Build history of the part. All positions in model axes, mm. Face numbers are marked on the shaded views. A direction names the side the tool comes from. Round coordinates to 2 decimals unless told otherwise and drop trailing zeros. Write each loop counter-clockwise with the first axis right and the second up, starting at its lowest first coordinate (ties: lowest second). Pieces come first, ordered by that corner, then holes. Notation, with made-up numbers: (87, 69.25) - (99, 69.25) arc R22 ccw to (99, 108.25) - close; hole circle Ø8 at (67.5, 6). An arc over 180 degrees is marked (long way). Write each question's results on one line, items separated by ' | '.
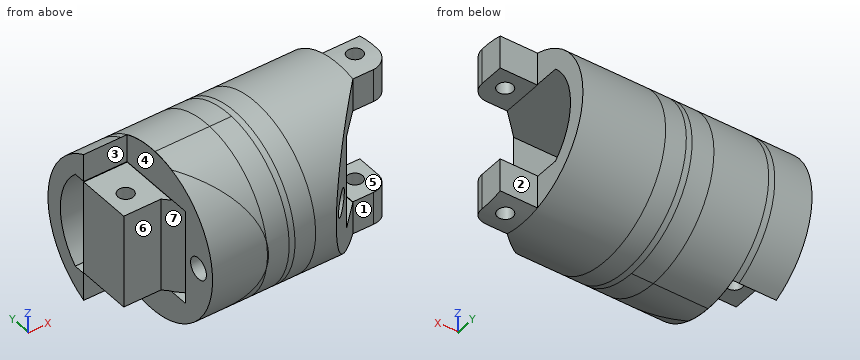
from build123d import *
from build123d.topology import SkipClean

# Parameters (mm, degrees)
SKETCH1_R           = 10
BOSS_EXTRUDE1_DEPTH = 10
SKETCH4_R           = 1.305
CUT_EXTRUDE3_DEPTH  = 25.5
BOSS_EXTRUDE2_START = 4.5
BOSS_EXTRUDE2_DEPTH = 4.5
SKETCH6_R           = 0.935
CUT_EXTRUDE4_DEPTH  = 12.25
SKETCH7_W           = 11.364916732
SKETCH7_H           = 5
BOSS_EXTRUDE3_DEPTH = 4.5
SKETCH8_R           = 0.935
CUT_EXTRUDE5_DEPTH  = 7.25
BOSS_EXTRUDE4_DEPTH = 4.5
CUT_EXTRUDE6_START  = -0.75
CUT_EXTRUDE6_DEPTH  = 0.75
SKETCH12_W          = 5.25
SKETCH12_H          = 4
CUT_EXTRUDE7_DEPTH  = 1.6
CUT_EXTRUDE8_DEPTH  = 15.8
FILLET1_R           = 2
CUT_EXTRUDE9_DEPTH  = 10.8
SKETCH15_W          = 11.364916732
SKETCH15_H          = 6.6
CUT_EXTRUDE10_DEPTH = 1.6
CUT_EXTRUDE11_DEPTH = 15
BOSS_EXTRUDE5_REACH = 35.438
SKETCH17_R          = 10
SKETCH17_R_2        = 1.305
CUT_EXTRUDE12_DEPTH = 14
SCALE1_SCALE        = 0.8


with BuildPart() as part:
    # Sketch1 → Boss-Extrude1 (new, symmetric)
    with BuildSketch(Plane(origin=(0, 0, 0), x_dir=(0, 0, -1), z_dir=(1, 0, 0))):
        Circle(SKETCH1_R)
    extrude(amount=BOSS_EXTRUDE1_DEPTH, both=True)

    # Sketch4 → Cut-Extrude3 (cut, symmetric)
    with BuildSketch(Plane(origin=(0, -0.76336978, 0), x_dir=(0, 0, -1), z_dir=(1, 0, 0))):
        with Locations((0, -6.913267104)):
            Circle(SKETCH4_R)
    extrude(amount=CUT_EXTRUDE3_DEPTH, both=True, mode=Mode.SUBTRACT)

    # Sketch5 → Boss-Extrude2 (add)
    with BuildSketch(Plane(origin=(10, 0, 0), x_dir=(0, 0, -1), z_dir=(1, 0, 0)).offset(BOSS_EXTRUDE2_START)):
        with BuildLine():
            Line((-9.682458366, -2.5), (-5.682458366, -2.5))
            Line((-5.682458366, -2.5), (-5.682458366, 2.5))
            Line((-5.682458366, 2.5), (-9.682458366, 2.5))
            ThreePointArc((-9.682458366, 2.5), (-10, 0), (-9.682458366, -2.5))
        make_face()
    boss_extrude2 = extrude(amount=-BOSS_EXTRUDE2_DEPTH)

    # Mirror1: Boss-Extrude2 across plane
    add(boss_extrude2.mirror(Plane.XY))

    # Sketch6 → Cut-Extrude4 (cut, symmetric)
    with SkipClean():  # the faces are left unmerged after this step: merging them gives an invalid solid
        with BuildSketch(Plane.XY):
            with Locations((12.25, 0.25)):
                Circle(SKETCH6_R)
        extrude(amount=CUT_EXTRUDE4_DEPTH, both=True, mode=Mode.SUBTRACT)

    # Sketch7 → Boss-Extrude3 (add)
    with SkipClean():  # the faces are left unmerged after this step: merging them gives an invalid solid
        with BuildSketch(Plane.ZY.offset(10)):
            Rectangle(SKETCH7_W, SKETCH7_H)
        extrude(amount=BOSS_EXTRUDE3_DEPTH)

    # Sketch8 → Cut-Extrude5 (cut, symmetric)
    with SkipClean():  # the faces are left unmerged after this step: merging them gives an invalid solid
        with BuildSketch(Plane.XY):
            with Locations((-12.25, 0.25)):
                Circle(SKETCH8_R)
        extrude(amount=CUT_EXTRUDE5_DEPTH, both=True, mode=Mode.SUBTRACT)

    # Sketch10 → Boss-Extrude4 (add)
    with SkipClean():  # the faces are left unmerged after this step: merging them gives an invalid solid
        with BuildSketch(Plane.ZY.offset(10)):
            with BuildLine():
                Line((9.682458366, 2.5), (-9.682458366, 2.5))
                ThreePointArc((-9.682458366, 2.5), (0, 10), (9.682458366, 2.5))
            make_face()
        extrude(amount=BOSS_EXTRUDE4_DEPTH)

    # Cut-Extrude6: read off the stored shape, not the designer's step
    # Cut-Extrude6 outline → Cut-Extrude6 (cut)
    with SkipClean():  # the faces are left unmerged after this step: merging them gives an invalid solid
        with BuildSketch(Plane.ZY.offset(10).offset(CUT_EXTRUDE6_START)):
            with BuildLine():
                ThreePointArc((-9.682458366, 2.5), (-9.369942303, -3.493448331), (-5.682458366, -8.228588392))
                Line((-5.682458366, -8.228588392), (-5.682458366, 2.5))
                Line((-5.682458366, 2.5), (-9.682458366, 2.5))
            make_face()
            with BuildLine():
                Line((5.682458366, 2.5), (5.682458366, -8.228588392))
                ThreePointArc((5.682458366, -8.228588392), (9.369942303, -3.493448331), (9.682458366, 2.5))
                Line((9.682458366, 2.5), (5.682458366, 2.5))
            make_face()
        extrude(amount=CUT_EXTRUDE6_DEPTH, mode=Mode.SUBTRACT)

    # Sketch12 → Cut-Extrude7 (cut)
    with SkipClean():  # the faces are left unmerged after this step: merging them gives an invalid solid
        with BuildSketch(Plane.XZ.offset(-2.5)):
            with Locations((-11.875, -7.682458366)):
                Rectangle(SKETCH12_W, SKETCH12_H)
            with Locations((-11.875, 7.682458366)):
                Rectangle(SKETCH12_W, SKETCH12_H)
        extrude(amount=-CUT_EXTRUDE7_DEPTH, mode=Mode.SUBTRACT)

    # Sketch13 → Cut-Extrude8 (cut, symmetric)
    with SkipClean():  # the faces are left unmerged after this step: merging them gives an invalid solid
        with BuildSketch(Plane.XY):
            Polygon((-10, -8.228588392), (-10, -2.5), (-2.5, -10), (-10, -10), align=None)
        extrude(amount=CUT_EXTRUDE8_DEPTH, both=True, mode=Mode.SUBTRACT)

    # Fillet1
    fillet1_edges = [part.edges().sort_by_distance(p)[0] for p in [
        (14.5, -2.5, 7.682458366),
        (14.5, -2.5, -7.682458366),
    ]]
    fillet(fillet1_edges, radius=FILLET1_R)

    # Sketch14 → Cut-Extrude9 (cut, symmetric)
    with SkipClean():  # the faces are left unmerged after this step: merging them gives an invalid solid
        with BuildSketch(Plane.XY):
            Polygon((10, -10), (10, -2.5), (2.5, -10), align=None)
        extrude(amount=CUT_EXTRUDE9_DEPTH, both=True, mode=Mode.SUBTRACT)

    # Sketch15 → Cut-Extrude10 (cut)
    with SkipClean():  # the faces are left unmerged after this step: merging them gives an invalid solid
        with BuildSketch(Plane(origin=(10, 0, 0), x_dir=(0, 0, -1), z_dir=(1, 0, 0))):
            with Locations((0, -0.8)):
                Rectangle(SKETCH15_W, SKETCH15_H)
        extrude(amount=-CUT_EXTRUDE10_DEPTH, mode=Mode.SUBTRACT)

    # Sketch16 → Cut-Extrude11 (cut)
    with SkipClean():  # the faces are left unmerged after this step: merging them gives an invalid solid
        with BuildSketch(Plane(origin=(10, 0, 0), x_dir=(0, 0, -1), z_dir=(1, 0, 0))):
            with BuildLine():
                Line((-5.75, 5.5), (-5.75, -5.5))
                Line((-5.75, -5.5), (5.75, -5.5))
                Line((5.75, -5.5), (5.75, 5.5))
                ThreePointArc((5.75, 5.5), (0, 7.956915231), (-5.75, 5.5))
            make_face()
        extrude(amount=-CUT_EXTRUDE11_DEPTH, mode=Mode.SUBTRACT)


with BuildPart() as body_2:
    # Split1: the piece on the far side of the plane
    add(part.part)
    split(bisect_by=Plane(origin=(0, 0, 0), x_dir=(0, 0, 1), z_dir=(1, 0, 0)), keep=Keep.BOTTOM)


with BuildPart() as part_1:
    add(part.part)

    # Split1
    split(bisect_by=Plane(origin=(0, 0, 0), x_dir=(0, 0, 1), z_dir=(1, 0, 0)), keep=Keep.TOP)


with BuildPart() as part_2:
    # Body-Move/Copy1: moved
    add(part_1.part.moved(Location((15.8, 0, 0))))


    # Sketch17 → Boss-Extrude5 (add, up to next)
    with BuildSketch(Plane.ZY.offset(-15.8), mode=Mode.PRIVATE) as boss_extrude5_sk1:
        with Locations(Location((0, 0, 0), (0, 0, 357.134016017))):
            Circle(SKETCH17_R)
        with Locations(Location((0, -7.676636884, 0), (0, 0, 180))):
            Circle(SKETCH17_R_2, mode=Mode.SUBTRACT)
        with BuildLine():
            Line((-5.75, -5.5), (5.75, -5.5))
            Line((5.75, -5.5), (5.75, 5.5))
            ThreePointArc((5.75, 5.5), (0, 7.956915231), (-5.75, 5.5))
            Line((-5.75, 5.5), (-5.75, -5.5))
        make_face(mode=Mode.SUBTRACT)
    boss_extrude5_tool1 = extrude(boss_extrude5_sk1.sketch, amount=BOSS_EXTRUDE5_REACH, mode=Mode.PRIVATE) - body_2.part
    add(boss_extrude5_tool1.solids().sort_by_distance((15.8, 0.485858, -9.705003))[0])


with BuildPart() as body_2_1:
    # Body-Move/Copy2: moved
    add(body_2.part.moved(Location((9.26, 0, 0))))

    # Combine4: union part
    add(part_2.part)

    # Sketch18 → Cut-Extrude12 (cut)
    with SkipClean():  # the faces are left unmerged after this step: merging them gives an invalid solid
        with BuildSketch(Plane.ZY.offset(5.24)):
            with BuildLine():
                Line((-5.75, 5.5), (-5.75, 4.1))
                Line((-5.75, 4.1), (5.75, 4.1))
                Line((5.75, 4.1), (5.75, 5.5))
                ThreePointArc((5.75, 5.5), (0, 7.956915231), (-5.75, 5.5))
            make_face()
        extrude(amount=-CUT_EXTRUDE12_DEPTH, mode=Mode.SUBTRACT)


with BuildPart() as body_2_2:
    # Scale1: scaled about (10.157754057, 0.26372377, 1.86e-07)
    add(body_2_1.part.scale(SCALE1_SCALE).moved(Location((2.031550811, 0.052744754, 3.7e-08))))


with BuildPart() as body_2_2_1:
    # Split2: the piece on the far side of the plane
    add(body_2_2.part)
    split(bisect_by=Plane(origin=(10, 0, 0), x_dir=(0, 0, 1), z_dir=(1, 0, 0)), keep=Keep.BOTTOM)


with BuildPart() as body_2_3:
    add(body_2_2.part)

    # Split2
    split(bisect_by=Plane(origin=(10, 0, 0), x_dir=(0, 0, 1), z_dir=(1, 0, 0)), keep=Keep.TOP)


with BuildPart() as body_2_4:
    # Body-Move/Copy3: read off the stored shape, not the designer's step
    # Body-Move/Copy3: moved
    add(body_2_3.part.moved(Location((-2.6715551, 0, 0))))


with BuildPart() as body_2_2_2:
    add(body_2_2_1.part)

    # Combine5: union body 2
    add(body_2_4.part)


solid = body_2_2_2.part
(1) Flat gauge pins, fed straight in: pin 1 Ø0.5 at (x, y) = (3, -0.5) entering from -Z; pin 2 Ø4.5 at (x, y) = (-1, 0.5) entering from +Z; pin 3 Ø4 at (y, z) = (-4, 3) entering from -X. Where does each tip first touch, or does it go through?
Worked answers:
pin 1: stops at z = -7.99 | pin 2: stops at z = 4.55 | pin 3: stops at x = 1.49
(2) Tool access for the marked faces 1, 2, 3, 4 and 5: list every direction of +Z, -Z, +X, -X, +Y, -Y with a clear straight run to the whole face (end or side of a thin tool).
Worked answers:
face 1: +Z, -Z, +X, -Y | face 2: +Z, -Z, +X, +Y | face 3: +Z, -X, -Y | face 4: -X, -Y | face 5: +X, +Y, -Y
(3) Drill centre lines: probe 1 along Z at (x, y) = (20.5, 0.5); probe 2 along Y at (x, z) = (10.25, 0.75); probe 3 along X at (y, z) = (-0.25, 5.5). Where is each one in solid material? Low to high. Write a range as [from, to].
Worked answers:
probe 1: z = [-7.99, -4.55], [4.55, 7.99] | probe 2: y = [-7.91, -6.81], [-5.36, -4.35], [6.37, 8.02] | probe 3: x = [2.03, 21.25], [22.35, 23.6]
(4) Slice it at C-C, the plane z = -3. Write the cut outline in (x, y), and give its area (3 significant figures).
Worked answers:
outline: (-2.16, -1.95) - (1.44, -1.95) - (3.84, -4.35) - (2.03, -4.35) - (2.03, -7.36) - (14.58, -7.36) - (17.6, -4.35) - (5.44, -4.35) - (5.44, 3.33) - (-2.16, 3.33) - close; (-2.16, 5.67) - (20, 5.67) - (20, 7.47) - (-2.16, 7.47) - close; hole circle Ø1.5 at (-0.36, 0.25) | area: 127 mm2
(5) Slice it at B-B, the plane y = 5.75. Write the cut outline in (x, z).
Worked answers:
outline: (-2.16, -5.62) - (20, -5.62) - (20, -2.84) - (-2.16, -2.84) - close; (-2.16, 2.84) - (20, 2.84) - (20, 5.62) - (-2.16, 5.62) - close
(6) Slice it at A-A, the plane z = 0. Write the cut outline in (x, y).
Worked answers:
outline: (-2.16, -1.95) - (1.44, -1.95) - (3.84, -4.35) - (2.03, -4.35) - (2.03, -5.04) - (16.9, -5.04) - (17.6, -4.35) - (5.44, -4.35) - (5.44, 3.33) - (-2.16, 3.33) - close; (-2.16, 6.42) - (20, 6.42) - (20, 8.05) - (-2.16, 8.05) - close; (2.03, -7.95) - (14, -7.95) - (14.81, -7.13) - (2.03, -7.13) - close; hole circle Ø1.5 at (-0.36, 0.25)
(7) Two-plate mould, pull along Z, no slides. Class the marked faces 6 and 7: released by +Z, released by -Z, zero draft, split by the parting line, or undercut.
Worked answers:
face 6: zero draft | face 7: undercut
(8) Slice it at D-D, the plane z = -6. Write the cut outline in (x, y), and give its area (3 significant figures).
Worked answers:
outline: (-2.16, 3.33) - (2.03, 3.33) - (2.03, -5.24) - (16.71, -5.24) - (20, -1.95) - (22, -1.95) arc R1.6 ccw to (23.6, -0.35) - (23.6, 2.05) - (20, 2.05) - (20, 5.34) - (-2.16, 5.34) - close; hole circle Ø1.5 at (21.8, 0.25) | area: 205 mm2
